Study the drawing (mm; zero at the part's minimum x, y, z) and answer. Give positions to 0.01 mm unless a question says otherwise; leave off trailing zeros. Order: outer loops, then holes, each group sorted by start corner. A loop starts at its lowest first (then second) coordinate and runs counter-clockwise, first axis right, second up.
Item 1: Find the intervals of material crossed by line 1 along Z through (x, y) = (3, 1.05); line 2 along Z through (x, y) = (3.9, 1.35); line 3 along X through (y, z) = (0.9, 21), in increasing order.
Item 2: A cutting plane is placed at B-B (y = 0.35). Write down the section's boundary in (x, z).
Item 3: Given pin 1 Ø2 at (x, z) = (1, 11.5) entering from -Y, flat-ended and moving along its own axis, determine where the tip first touches the part or whether it passes through.
Item 4: A cutting plane is placed at C-C (x = 1.85). Write down the section's boundary in (y, z), plus the area to 3 significant figures.
Item 5: A cutting plane is placed at A-A (x = 3). Write down the section's boundary in (y, z), plus the area to 3 significant figures.
Item 6: A cutting plane is placed at D-D (x = 5.55). Write down the section's boundary in (y, z), plus the area to 3 significant figures.
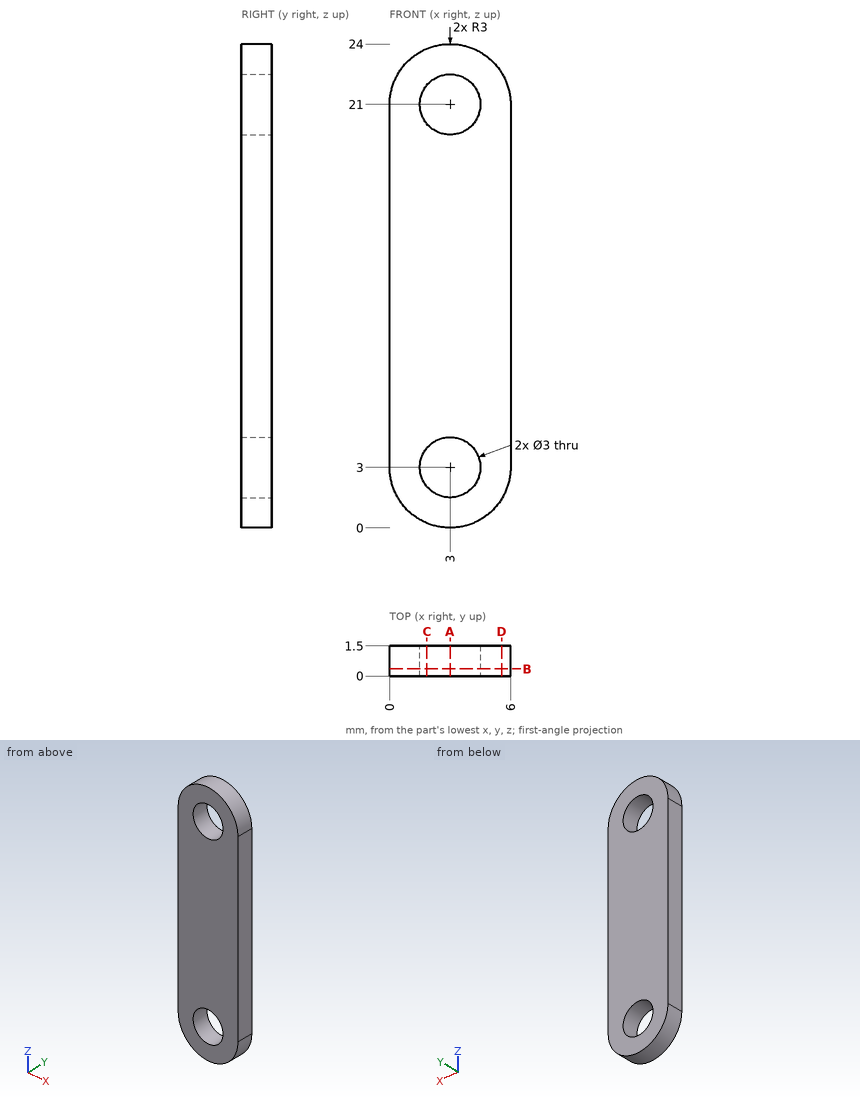
Response values:
1. line 1: z = 0 to 1.5, 4.5 to 19.5, 22.5 to 24
1. line 2: z = 0.14 to 1.8, 4.2 to 19.8, 22.2 to 23.86
1. line 3: x = 0 to 1.5, 4.5 to 6
2. outline: (0, 3) arc R3 ccw to (6, 3) - (6, 21) arc R3 ccw to (0, 21) - close; hole circle Ø3 at (3, 3); hole circle Ø3 at (3, 21)
3. pin 1: stops at y = 0
4. outline: (0, 0.23) - (1.5, 0.23) - (1.5, 2.04) - (0, 2.04) - close; (0, 3.96) - (1.5, 3.96) - (1.5, 20.04) - (0, 20.04) - close; (0, 21.96) - (1.5, 21.96) - (1.5, 23.77) - (0, 23.77) - close
4. area: 29.5 mm2
5. outline: (0, 0) - (1.5, 0) - (1.5, 1.5) - (0, 1.5) - close; (0, 4.5) - (1.5, 4.5) - (1.5, 19.5) - (0, 19.5) - close; (0, 22.5) - (1.5, 22.5) - (1.5, 24) - (0, 24) - close
5. area: 27.0 mm2
6. outline: (0, 1.42) - (1.5, 1.42) - (1.5, 22.58) - (0, 22.58) - close
6. area: 31.7 mm2
